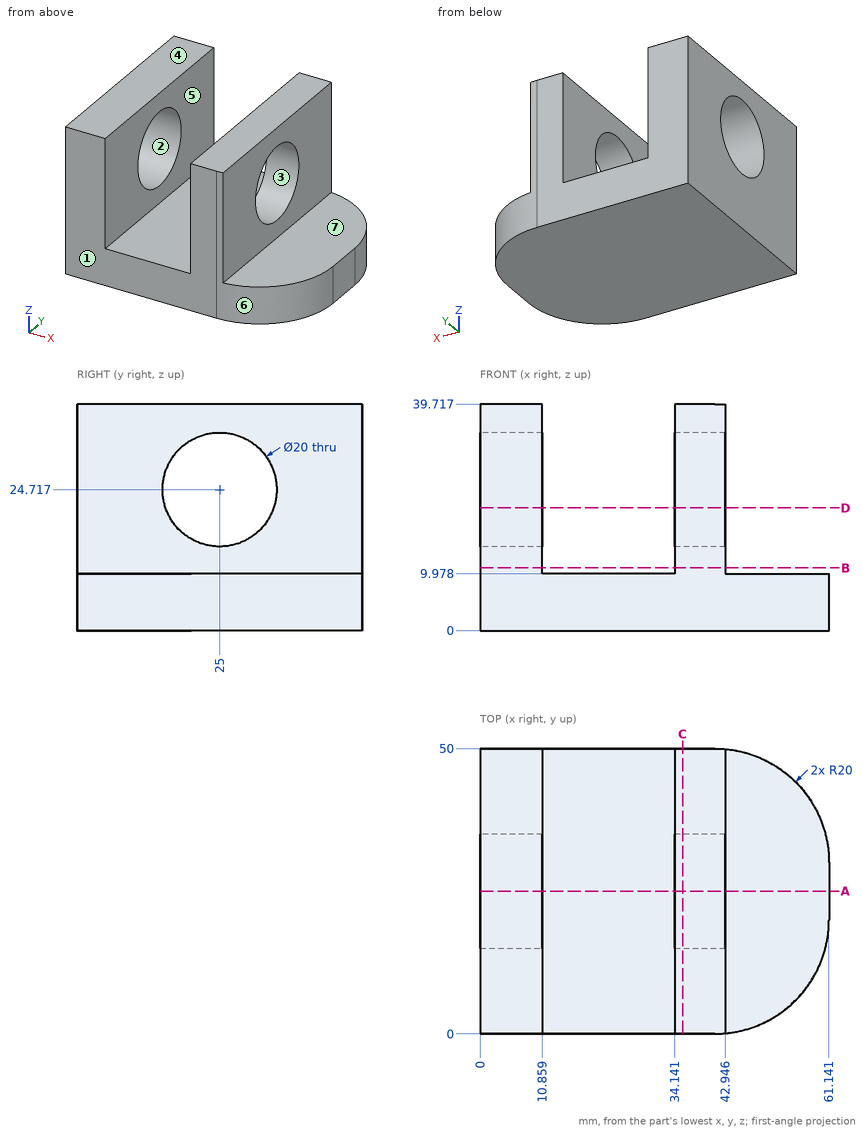
Could you check a few things on this drawing? It's one solid part, dimensions in mm from its lowest x, y, z. A direction names the side the tool comes from. Give positions to 0.01 mm unless a question says otherwise; leave off trailing zeros. Write each loop counter-clockwise with the first axis right and the second up, starting at its lowest first coordinate (ties: lowest second). Pieces come first, ordered by that corner, then holes. Notation, with made-up numbers: M 82,34.25 L 138,34.25 A22 ccw 138,69.25 Z; hole C 8,89 d6. An arc over 180 degrees is marked long. Put each result on its own line as item: value. Start each with the question number.
Item 1: On a 3-axis mill with a long thin cutter (end or side, diameter ignored), from which of +Z, -Z, +X, -X, +Y, -Y can I reach the whole of each face in a straight line? I mean the marked faces 5, 6 and 7. Say none if no direction works.
Item 2: Thinking about a two-plate mould opening in Z: for the marked faces 1, 2, 3 and 4, which applies, +Z half, -Z half, draft (parallel to the pull), parting line (faces both ways), or undercut?
Item 3: If we section it at C-C, the plane x = 35.5: Write out the boundary of the cut face in (y, z).
Item 4: Will these pins go through, and if not, where does the flat tip stop? pin 1 (4 mm diameter, centred on x = 23.5, y = 6.5, fed in from +Z); pin 2 (23 mm diameter, centred on y = 25, z = 24.72, fed in from +X); pin 3 (5 mm diameter, centred on x = 46, z = 9.5, fed in from +Y).
Item 5: If we section it at A-A, the plane y = 25: Write out the boundary of the cut face in (x, z) (1 decimal).
Item 6: I need wall thicknesses on L1, parallel to Z at x = 37.75, y = 25; L2, parallel to X at y = 4, z = 34 (1 decimal); L3, parallel to Z at x = 54.5, y = 12. Which ranges of each line are inside material? Lowest first, please. Write a range as from..to.
Item 7: If we section it at D-D, the plane z = 21.5: Write out the boundary of the cut face in (x, y) (1 decimal).
Item 8: If we section it at B-B, the plane z = 11: Write out the boundary of the cut face in (x, y) (1 decimal).
Values:
1. face 5: +Z, +Y, -Y
1. face 6: +Z, -Z, +X, -Y
1. face 7: +Z, +X, +Y, -Y
2. face 1: draft
2. face 2: undercut
2. face 3: undercut
2. face 4: +Z half
3. outline: M 0,0 L 50,0 L 50,39.72 L 0,39.72 Z; hole C 25,24.72 d20
4. pin 1: z = 9.98
4. pin 2: x = 42.95
4. pin 3: y = 49.86
5. outline: M 0,0 L 61.1,0 L 61.1,10 L 42.9,10 L 42.9,14.7 L 34.1,14.7 L 34.1,10 L 10.9,10 L 10.9,14.7 L 0,14.7 Z; M 0,34.7 L 10.9,34.7 L 10.9,39.7 L 0,39.7 Z; M 34.1,34.7 L 42.9,34.7 L 42.9,39.7 L 34.1,39.7 Z
6. L1: 0..14.72, 34.72..39.72
6. L2: 0..10.9, 34.1..42.9
6. L3: 0..9.98
7. outline: M 0,0 L 10.9,0 L 10.9,15.5 L 0,15.5 Z; M 0,34.5 L 10.9,34.5 L 10.9,50 L 0,50 Z; M 34.1,0 L 41.1,0 A20 ccw 42.9,0.1 L 42.9,15.5 L 34.1,15.5 Z; M 34.1,34.5 L 42.9,34.5 L 42.9,49.9 A20 ccw 41.1,50 L 34.1,50 Z
8. outline: M 0,0 L 10.9,0 L 10.9,50 L 0,50 Z; M 34.1,0 L 41.1,0 A20 ccw 42.9,0.1 L 42.9,49.9 A20 ccw 41.1,50 L 34.1,50 Z
